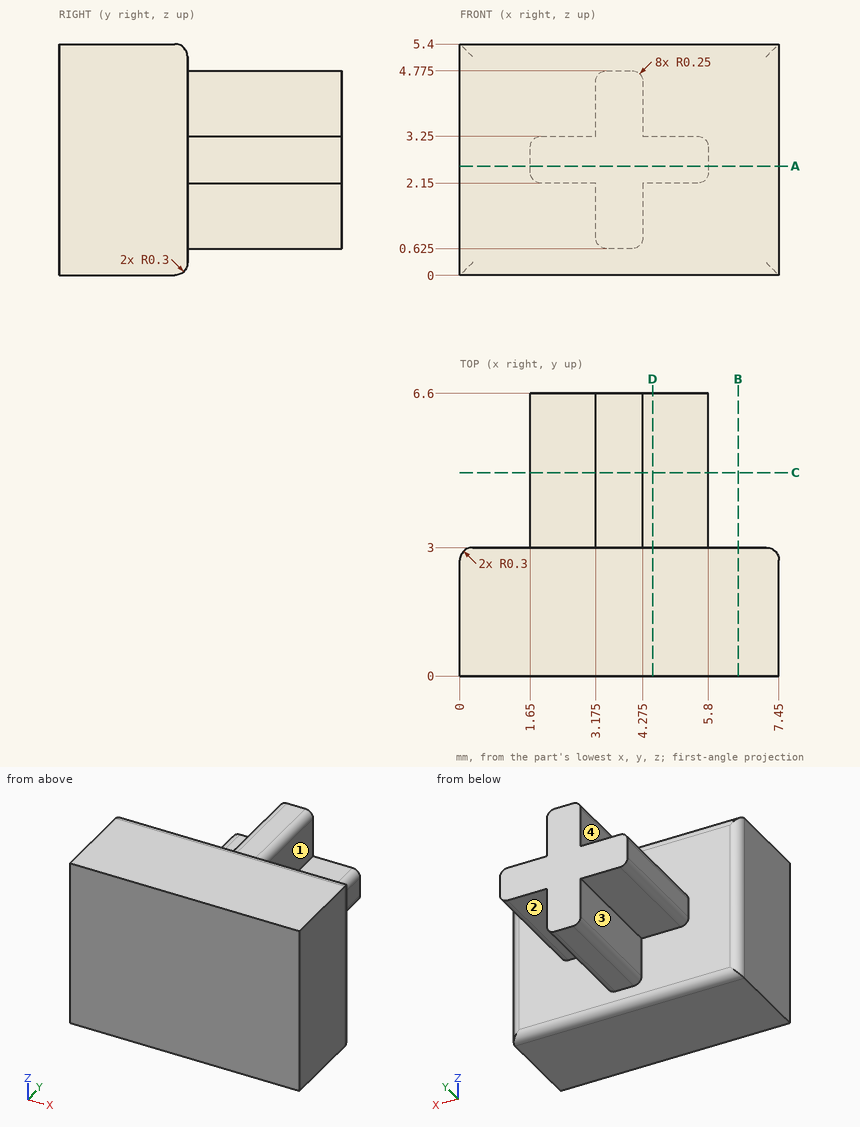
Job drawing, mm, ordinate dimensions from the low corner. One solid piece. A direction names the side the tool comes from. Round coordinates to 2 decimals unless told otherwise and drop trailing zeros. Loops run counter-clockwise (first coordinate to the right, second up) from the corner with the lowest first, then second, coordinate; pieces in that order, holes last.
(1) Which spindle directions (+Z, -Z, +X, -X, +Y, -Y) get a long thin tool onto all of the face, cutting with end or side? Do the marked faces 1, 2, 3 and 4. Say none if no direction does.
(2) Cut at C-C (y = 4.75). Give the cut face in (x, z) (3 decimals).
(3) Drop flat-ended pins along their axis: pin 1 (1 mm diameter, centred on y = 4.5, z = 3.5, fed in from -X); pin 2 (1 mm diameter, centred on y = 4.5, z = 1.5, fed in from -X) (3 decimals); pin 3 (1 mm diameter, centred on x = 4.5, y = 4.5, fed in from -Z) (3 decimals); pin 4 (3 mm diameter, centred on x = 6, z = 2, fed in from -Y). Give the stop position or say it passes through.
(4) Cut at B-B (x = 6.5). Give the cut face in (y, z), plus the area to 3 significant figures.
(5) Cut at A-A (z = 2.55). Give the cut face in (x, y).
(6) Cut at D-D (x = 4.5). Give the cut face in (y, z), plus the area to 3 significant figures.
(7) Wall check: line 1 along Y through (x, z) = (1.75, 1.1); line 2 along X through (y, z) = (5.5, 0.85); line 3 along Z through (x, y) = (4.5, 4.75). Give the ranges that are in metal, low to high.
Findings below:
1. face 1: +Z, +X, +Y
1. face 2: -Z, +X, +Y
1. face 3: -Z, -X, +Y
1. face 4: +Z, -X, +Y
2. outline: (1.65, 2.4) arc R0.25 ccw to (1.9, 2.15) - (3.175, 2.15) - (3.175, 0.875) arc R0.25 ccw to (3.425, 0.625) - (4.025, 0.625) arc R0.25 ccw to (4.275, 0.875) - (4.275, 2.15) - (5.55, 2.15) arc R0.25 ccw to (5.8, 2.4) - (5.8, 3) arc R0.25 ccw to (5.55, 3.25) - (4.275, 3.25) - (4.275, 4.525) arc R0.25 ccw to (4.025, 4.775) - (3.425, 4.775) arc R0.25 ccw to (3.175, 4.525) - (3.175, 3.25) - (1.9, 3.25) arc R0.25 ccw to (1.65, 3) - close
3. pin 1: stops at x = 1.65
3. pin 2: stops at x = 3.175
3. pin 3: stops at z = 0.625
3. pin 4: stops at y = 0
4. outline: (0, 0) - (2.7, 0) arc R0.3 ccw to (3, 0.3) - (3, 5.1) arc R0.3 ccw to (2.7, 5.4) - (0, 5.4) - close
4. area: 16.2 mm2
5. outline: (0, 0) - (7.45, 0) - (7.45, 2.7) arc R0.3 ccw to (7.15, 3) - (5.8, 3) - (5.8, 6.6) - (1.65, 6.6) - (1.65, 3) - (0.3, 3) arc R0.3 ccw to (0, 2.7) - close
6. outline: (0, 0) - (2.7, 0) arc R0.3 ccw to (3, 0.3) - (3, 2.15) - (6.6, 2.15) - (6.6, 3.25) - (3, 3.25) - (3, 5.1) arc R0.3 ccw to (2.7, 5.4) - (0, 5.4) - close
6. area: 20.1 mm2
7. line 1: y = 0 to 3
7. line 2: x = 3.18 to 4.27
7. line 3: z = 2.15 to 3.25
